from build123d import *

# Parameters (mm, degrees)
F0_W     = 900
F0_H     = 300
F1_DEPTH = 25
F2_W     = 850
F2_H     = 250
F3_DEPTH = 60


# Not quite as in the source:
# - a pattern or mirror of a feature is missing from the dataset's text; its kind, count and spacing are read off the source's solid


with BuildPart() as f1:
    # F0 (on Top) → F1 (new body)
    with BuildSketch(Plane.XY):
        Rectangle(F0_W, F0_H)
    extrude(amount=F1_DEPTH)


with BuildPart() as f1_copies_1:
    # F1_copies: instance of F1
    add(f1.part.mirror(Plane.XY.offset(55)))


with BuildPart() as f1_1:
    add(f1.part)

    add(f1_copies_1.part)  # F3 merges F1_copies_1
    # F2 (on face) → F3 (join)
    with BuildSketch(Plane.XY.offset(25)):
        Rectangle(F2_W, F2_H)
    extrude(amount=F3_DEPTH)


solid = f1_1.part
Geometry check sheet. Reference: the model listing, model coordinates, mm. A direction names the side the tool comes from. Give positions to 0.01 mm unless a question says otherwise; leave off trailing zeros. Order: outer loops, then holes, each group sorted by start corner. A loop starts at its lowest first (then second) coordinate and runs counter-clockwise, first axis right, second up. Notation, with made-up numbers: (74, 67) - (116, 67) arc R13 cw to (116, 82) - close; hole circle Ø6 at (68, 64.5). An arc over 180 degrees is marked (long way). Answer as a JSON object with one key per item and string values.
(1) Draft check along Z on faces 5 (the flat face through (425, -2, 55)), 6 (the flat face through (-6, 2, 110)), 7 (the flat face through (-6, 2, 0)), 8 (the flat face through (-35, -133, 25)). Enter one of: released by +Z, released by -Z, zero draft, split by the parting line, or undercut.
Report:
{"face 5": "undercut", "face 6": "released by +Z", "face 7": "released by -Z", "face 8": "undercut"}
(2) Cross-section at C-C (z = 35.5). Record the cut outline in (x, y).
Report:
{"outline": "(-425, -125) - (425, -125) - (425, 125) - (-425, 125) - close"}
(3) Tool access check on faces 1 (the flat face through (-6, -125, 55)), 2 (the flat face through (-425, -2, 55)), 3 (the flat face through (-35, -133, 85)), 4 (the flat face through (-6, 125, 55)). Record the directions out of +Z, -Z, +X, -X, +Y, -Y that give a thin tool (end or side, any length) a straight path to the whole face; none if there is none.
Report:
{"face 1": "+X, -X, -Y", "face 2": "-X, +Y, -Y", "face 3": "none", "face 4": "+X, -X, +Y"}
(4) Cross-section at B-B (y = 31.5). Record the cut outline in (x, z).
Report:
{"outline": "(-450, 0) - (450, 0) - (450, 25) - (425, 25) - (425, 85) - (450, 85) - (450, 110) - (-450, 110) - (-450, 85) - (-425, 85) - (-425, 25) - (-450, 25) - close"}
(5) Material ranges on line 1 (Y direction, x = 360.5, z = 46); line 2 (X direction, y = -113.5, z = 40.5), recorded low to high.
Report:
{"line 1": "-125 to 125", "line 2": "-425 to 425"}
(6) Depth check by flat-ended pin: pin 1 Ø1.5 at (y, z) = (-120, 47) entering from -X; pin 2 Ø5 at (x, z) = (31.5, 66.5) entering from -Y; pin 3 Ø6 at (x, z) = (256, 65) entering from +Y. Enter the tip coordinate at first touch or a pass-through.
Report:
{"pin 1": "x = -425", "pin 2": "y = -125", "pin 3": "y = 125"}
(7) Cross-section at A-A (x = -268). Record the cut outline in (y, z), then the cut area to 3 significant figures.
Report:
{"outline": "(-150, 0) - (150, 0) - (150, 25) - (125, 25) - (125, 85) - (150, 85) - (150, 110) - (-150, 110) - (-150, 85) - (-125, 85) - (-125, 25) - (-150, 25) - close", "area": "30,000 mm^2"}
